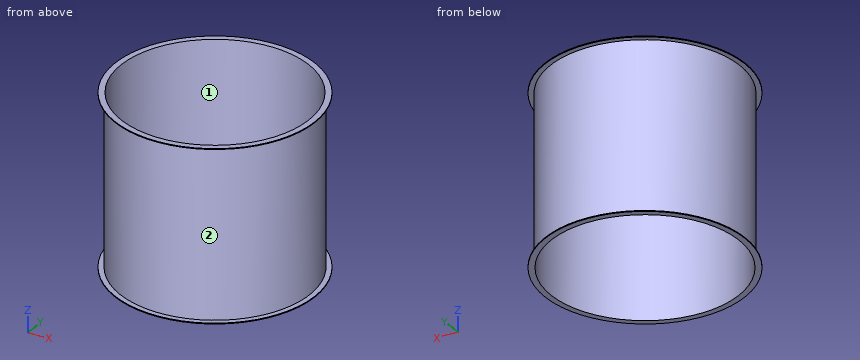
from build123d import *


with BuildPart() as f1:
    # F0 (on Front) → F1 (revolve)
    with BuildSketch(Plane.XZ):
        Polygon((-110, 0), (-110, 100), (-117, 100), (-117, 99), (-111, 99), (-111, 0), align=None)
        Polygon((-110, -100), (-110, 0), (-111, 0), (-111, -99), (-117, -99), (-117, -100), align=None)
    revolve(axis=Axis((0, 0, 50), (0, 0, -1)))


solid = f1.part
Part model, mm, in its own coordinate system. Face numbers are marked on the shaded views. Give positions to 0.01 mm unless a question says otherwise; leave off trailing zeros. Loops run counter-clockwise (first coordinate to the right, second up) from the corner with the lowest first, then second, coordinate; pieces in that order, holes last. Notation, with made-up numbers: M -19.5,-26 L 5.5,-26 A20 ccw 5.5,-14 Z; hole C 77.25,85.25 d1. An arc over 180 degrees is marked long. Put each result on its own line as item: value. Start each with the question number.
1) Saw through at A-A (y = 0). List the corners of the cut face in (x, z), then the cut area to 3 significant figures.
2) Flat gauge pins, fed straight in: pin 1 (12 mm diameter, centred on x = -63.5, y = -82.5, fed in from +Z); pin 2 (1 mm diameter, centred on x = 85, z = -34.5, fed in from -Y); pin 3 (10 mm diameter, centred on y = 7.5, z = -11.5, fed in from -X); pin 4 (1.5 mm diameter, centred on y = 25.5, z = 29.5, fed in from -X). Where does each tip first touch, or does it go through?
3) Probe probe 1 along Y at (x, z) = (0, -36); probe 2 along X at (y, z) = (-83, 19.5); probe 3 along Y at (x, z) = (-56, -74.5). List the from-to ranges inside material, lowest first.
4) Saw through at C-C (z = -26). List the corners of the cut face in (x, y), then the cut area to 3 significant figures.
5) Pull direction X, two halves, no side cores. Call the marked faces 1 and 2: +X half, -X half, draft (parallel to the pull), parting line (faces both ways), or undercut.
Numbers:
1. outline: M -117,-100 L -110,-100 L -110,100 L -117,100 L -117,99 L -111,99 L -111,-99 L -117,-99 Z; M 110,-100 L 117,-100 L 117,-99 L 111,-99 L 111,99 L 117,99 L 117,100 L 110,100 Z
1. area: 424 mm^2
2. pin 1: z = 100
2. pin 2: y = -71.98
2. pin 3: x = -110.97
2. pin 4: x = -108.21
3. probe 1: -111 to -110, 110 to 111
3. probe 2: -73.7 to -72.19, 72.19 to 73.7
3. probe 3: -95.84 to -94.68, 94.68 to 95.84
4. outline: C 0,0 d222; hole C 0,0 d220
4. area: 694 mm^2
5. face 1: undercut
5. face 2: parting line
